The listing builds one solid part. Answer for the finished solid, in the listing's coordinates (mm). Face numbers are marked on the shaded views. A direction names the side the tool comes from. Coordinates: 2 decimals unless noted, no trailing zeros. Write each loop counter-clockwise with the first axis right and the second up, starting at its lowest first coordinate (ties: lowest second). Pieces come first, ordered by that corner, then holes.
Autodesk Inventor part; units mm, degrees
ref_plane "YZ Plane" through (0, 0, 0) normal (1, 0, 0) x (0, 1, 0)
ref_plane "XZ Plane" through (0, 0, 0) normal (0, 1, 0) x (-1, 0, 0)
ref_plane "XY Plane" through (0, 0, 0) normal (0, 0, 1) x (1, 0, 0)
sketch "Sketch1" plane through (0, 0, 0) normal (0, 0, 1) x (1, 0, 0)
  line L0 (-33.02, 0) -> (-33.02, 50.8)
  line L1 (-33.02, 50.8) -> (0, 50.8)
  line L2 (0, 50.8) -> (0, 0)
  line L3 (-33.02, 0) -> (-26.67, 0)
  line L4 (-26.67, 0) -> (-26.67, 38.1)
  line L5 (-33.02, 50.8) -> (-33.02, 44.45)
  line L6 (-26.67, 38.1) -> (-6.35, 38.1)
  line L7 (0, 50.8) -> (-6.35, 50.8)
  line L8 (-6.35, 38.1) -> (-6.35, 0)
  line L9 (0, 0) -> (-6.35, 0)
  line L10 (-26.67, 0) -> (-33.02, 0)
  dimension "d0" = 33.02
  dimension "d1" = 50.8
  dimension "d2" = 6.35
  dimension "d3" = 6.35
  dimension "d4" = 6.35
  dimension "d11" = 50.8
  dimension "d15" = 38.1
extrude "Extrusion1" add sketch "Sketch1" along normal blind 25.4
sketch "Sketch2" plane through (0, 0, 0) normal (1, 0, 0) x (0, 0, -1)
  line L0 (0, 0) -> (-25.4, 0)
  line L1 (0, 50.8) -> (-25.4, 50.8)
  line L2 (-12.7, 0) -> (-12.7, 12.7)
  circle A0 centre (-12.7, 12.7) radius 6.35
  dimension "d7" = 12.7
  dimension "d8" = 12.7
extrude "Extrusion2" cut sketch "Sketch2" against normal blind 254
sketch "Sketch3" plane through (-33.02, 50.8, 0) normal (0, 1, 0) x (1, 0, 0)
  circle A0 centre (16.51, -12.7) radius 6.35
  dimension "d12" = 12.7
extrude "Extrusion3" add sketch "Sketch3" along normal blind 19.05
properties part number "small wheel support"
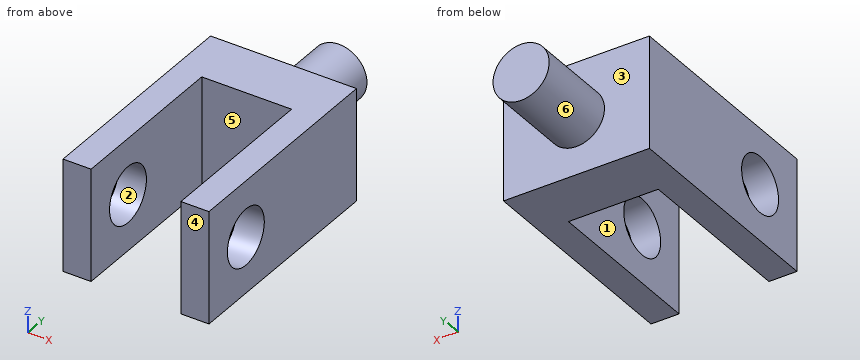
(1) Section D-D, the plane x = -3.5 is taken. Write down the section's boundary in (y, z).
(2) Section B-B, the plane z = 12.7 is taken. Write down the section's boundary in (x, y), plus the area to 3 significant figures.
(3) For a pull along Y with two mould halves and no side action, classify the marked faces 1, 2 and 3 as pulls with the +Y half, pulls with the -Y half, needs draft (parallel to the pull), parting line crosses it, or undercut.
(4) Section C-C, the plane y = 25.5 is taken. Write down the section's boundary in (x, z), plus the area to 3 significant figures.
(5) Which of the six approach directions +Z, -Z, +X, -X, +Y, -Y give full straight-line access (tool end or side, diameter ignored) to the marked faces 4, 5 and 6?
(6) Find the intervals of material crossed by probe 1 along X at (y, z) = (32.5, 4); probe 2 along Y at (x, z) = (-31.25, 12.7); probe 3 along Y at (x, z) = (-7, 3.25), in increasing order.
(7) Each of these flat-tipped pins is pushed along its axis until it touches: pin 1 (3 mm diameter, centred on x = -26, z = 22.5, fed in from +Y); pin 2 (3 mm diameter, centred on x = -22, z = 22, fed in from -Y); pin 3 (1.5 mm diameter, centred on y = 58, z = 16, fed in from +X). Where does it stop, or does it pass through?
(8) Section A-A, the plane y = 12.7 is taken. Write down the section's boundary in (x, z), plus the area to 3 significant figures.
Solution:
1. outline: (0, 0) - (50.8, 0) - (50.8, 25.4) - (0, 25.4) - close; hole circle Ø12.7 at (12.7, 12.7)
2. outline: (-33.02, 0) - (-26.67, 0) - (-26.67, 6.35) - (-33.02, 6.35) - close; (-33.02, 19.05) - (-26.67, 19.05) - (-26.67, 38.1) - (-6.35, 38.1) - (-6.35, 19.05) - (0, 19.05) - (0, 50.8) - (-10.16, 50.8) - (-10.16, 69.85) - (-22.86, 69.85) - (-22.86, 50.8) - (-33.02, 50.8) - close; (-6.35, 0) - (0, 0) - (0, 6.35) - (-6.35, 6.35) - close
2. area: 984 mm2
3. face 1: needs draft
3. face 2: undercut
3. face 3: pulls with the +Y half
4. outline: (-33.02, 0) - (-26.67, 0) - (-26.67, 25.4) - (-33.02, 25.4) - close; (-6.35, 0) - (0, 0) - (0, 25.4) - (-6.35, 25.4) - close
4. area: 323 mm2
5. face 4: +Z, -Z, +X, -X, -Y
5. face 5: +Z, -Z, -Y
5. face 6: +Y
6. probe 1: x = -33.02 to -26.67, -6.35 to 0
6. probe 2: y = 0 to 6.35, 19.05 to 50.8
6. probe 3: y = 38.1 to 50.8
7. pin 1: stops at y = 50.8
7. pin 2: stops at y = 38.1
7. pin 3: stops at x = -10.69
8. outline: (-33.02, 0) - (-26.67, 0) - (-26.67, 6.35) - (-33.02, 6.35) - close; (-33.02, 19.05) - (-26.67, 19.05) - (-26.67, 25.4) - (-33.02, 25.4) - close; (-6.35, 0) - (0, 0) - (0, 6.35) - (-6.35, 6.35) - close; (-6.35, 19.05) - (0, 19.05) - (0, 25.4) - (-6.35, 25.4) - close
8. area: 161 mm2
